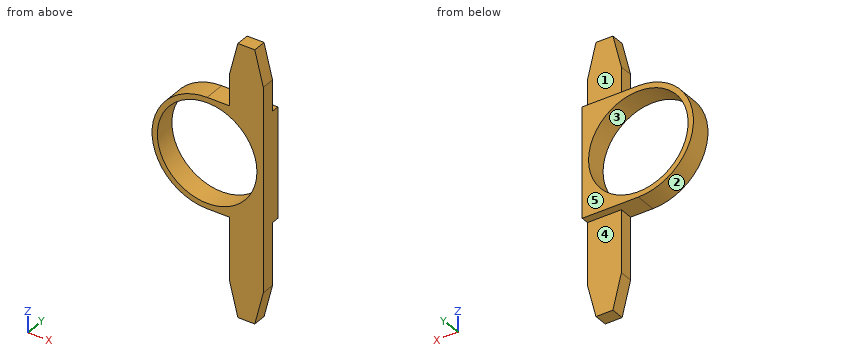
Autodesk Inventor part; units mm, degrees
ref_plane "YZ Plane" through (0, 0, 0) normal (1, 0, 0) x (0, 1, 0)
ref_plane "XZ Plane" through (0, 0, 0) normal (0, 1, 0) x (-1, 0, 0)
ref_plane "XY Plane" through (0, 0, 0) normal (0, 0, 1) x (1, 0, 0)
sketch "Sketch1" plane through (0, 0, 0) normal (0, 1, 0) x (-1, 0, 0)
  line L0 (0.8, 12.8) -> (-0.8, 12.8)
  line L1 (-1.6, 9.6) -> (-1.6, -9.6)
  line L2 (-0.8, -12.8) -> (0.8, -12.8)
  line L3 (1.6, -9.6) -> (1.6, 9.6)
  line L4 (1.6, 9.6) -> (0.8, 12.8)
  line L5 (-1.6, 9.6) -> (-0.8, 12.8)
  line L6 (1.6, -9.6) -> (0.8, -12.8)
  line L7 (-1.6, -9.6) -> (-0.8, -12.8)
  line L8 (-1.6, 6.2) -> (-1.6, -4.2)
  point P0 (0, 0)
  point P1 (1.6, 12.8)
  point P2 (-1.6, 12.8)
  point P3 (1.6, -12.8)
  dimension "d0" = 25.6
  dimension "d1" = 3.2
  dimension "d2" = 1.6
  dimension "d3" = 12.8
  dimension "d4" = 3.2
  dimension "d12" = 0
extrude "Extrusion1" add sketch "Sketch1" along normal blind 1.27
sketch "Sketch4" plane through (0, 0, 0) normal (0, -1, 0) x (1, 0, 0)
  line L0 (1.6, -3.7217) -> (-3.7, -3.7217)
  line L1 (-3.7, 6.6783) -> (1.6, 6.6783)
  line L2 (1.6, 6.6783) -> (1.6, -3.7217)
  line L3 (1.6, 9.6) -> (1.6, -9.6)
  arc A0 (-3.7, 6.6783) -> (-3.7, -3.7217) centre (-3.7, 1.4783) ccw
  point P0 (0, 0)
  dimension "d23" = 10.4
  dimension "d24" = 0
  dimension "d27" = 5.3
extrude "Extrusion2" add sketch "Sketch4" against normal blind 2
sketch "Sketch5" plane through (0, 2, 0) normal (0, 1, 0) x (1, 0, 0)
  circle A0 centre (-3.7, -1.4783) radius 4.7
  line L0 (1.6, -6.6783) -> (1.6, 3.7217)
  line L1 (-3.7, -6.6783) -> (1.6, -6.6783)
  point P0 (0, 0)
  dimension "d30" = 9.4
  dimension "d31" = 5.3
  dimension "d32" = 5.2
extrude "Extrusion3" cut sketch "Sketch5" against normal blind 2
properties part number "Headbar_D_Shape_unfinished"
Work out the finished part from the listing and answer in its coordinate system (mm). Face numbers are marked on the shaded views. A direction names the side the tool comes from. Round coordinates to 2 decimals unless told otherwise and drop trailing zeros. Loops run counter-clockwise (first coordinate to the right, second up) from the corner with the lowest first, then second, coordinate; pieces in that order, holes last. Notation, with made-up numbers: M -14.5,-21 L 23.5,-21 A36 cw 23.5,17 Z; hole C 5.5,-14 d8. An arc over 180 degrees is marked long. One line per question, with ' | ' between items. Start each with the question number.
(1) A cutting plane is placed at C-C on y = 1.6. Write down the section's boundary in (x, z), plus the area to 3 significant figures.
(2) A tool of negligible diameter and unlimited length cuts with its end or side. For the marked faces 4 and 5, from which of +Z, -Z, +X, -X, +Y, -Y can it reach the whole face along a straight path? Write none if from no direction.
(3) A cutting plane is placed at B-B on x = -5.25. Write down the section's boundary in (y, z).
(4) For a pull along X with two mould halves and no side action, classify the marked faces 1, 2 and 3 as released by +X, released by -X, zero draft, split by the parting line, or undercut.
(5) Find the intervals of material crossed by line 1 (Z direction, x = -3.7, y = 1); line 2 (Y direction, x = -0.5, z = 7); line 3 (X direction, y = 1.95, z = -2.25), in increasing order.
(6) A cutting plane is placed at D-D on x = 0.5. Write down the section's boundary in (y, z), plus the area to 3 significant figures.
(7) Flat-ended cylindrical pins translate along their axes: pin 1 Ø5 at (x, z) = (-5.5, -9.5) entering from +Y (3 decimals); pin 2 Ø2.5 at (x, z) = (0.5, 8.5) entering from +Y; pin 3 Ø1 at (y, z) = (0.5, 8.5) entering from -X; pin 4 Ø1 at (y, z) = (1.5, -3.5) entering from -X. Find the tip coordinate at first contact, or state that the pin passes through.
(8) A cutting plane is placed at A-A on z = -2.75. Write down the section's boundary in (x, y), plus the area to 3 significant figures.
Geometry check:
1) outline: M -3.7,-3.72 L 1.6,-3.72 L 1.6,6.68 L -3.7,6.68 A5.2 ccw Z; hole C -3.7,1.48 d9.4 | area: 28.2 mm²
2) face 4: -Z, +X, -X, +Y | face 5: +Z, -Z, +X, -X, +Y
3) outline: M 0,-3.49 L 2,-3.49 L 2,-2.96 L 0,-2.96 Z; M 0,5.92 L 2,5.92 L 2,6.44 L 0,6.44 Z
4) face 1: zero draft | face 2: released by -X | face 3: undercut
5) line 1: z = -3.72 to -3.22, 6.18 to 6.68 | line 2: y = 0 to 1.27 | line 3: x = -7.32 to -6.56, -0.84 to 1.6
6) outline: M 0,-12.8 L 1.27,-12.8 L 1.27,-3.72 L 2,-3.72 L 2,-0.63 L 0,-0.63 Z; M 0,3.59 L 2,3.59 L 2,6.68 L 1.27,6.68 L 1.27,12.8 L 0,12.8 Z | area: 31.7 mm²
7) pin 1: passes through | pin 2: stops at y = 1.27 | pin 3: stops at x = -1.6 | pin 4: stops at x = -6.34
8) outline: M -6.73,0 L -5.75,0 L -5.75,2 L -6.73,2 Z; M -1.65,0 L 1.6,0 L 1.6,2 L -1.65,2 Z | area: 8.44 mm²
